Can you work these out from the drawing? Everything is in mm from the part's minimum corner. A direction names the side the tool comes from. Give positions to 0.01 mm unless a question says otherwise; leave off trailing zeros. Loops run counter-clockwise (first coordinate to the right, second up) from the corner with the lowest first, then second, coordinate; pieces in that order, holes last. Notation, with made-up numbers: (39.5, -6) - (85.5, -6) arc R14 ccw to (85.5, -1) - close; hole circle Ø9 at (-23.5, -3.5). An arc over 180 degrees is marked (long way). Write each question's results on one line, items separated by ' | '. Start each with the question number.
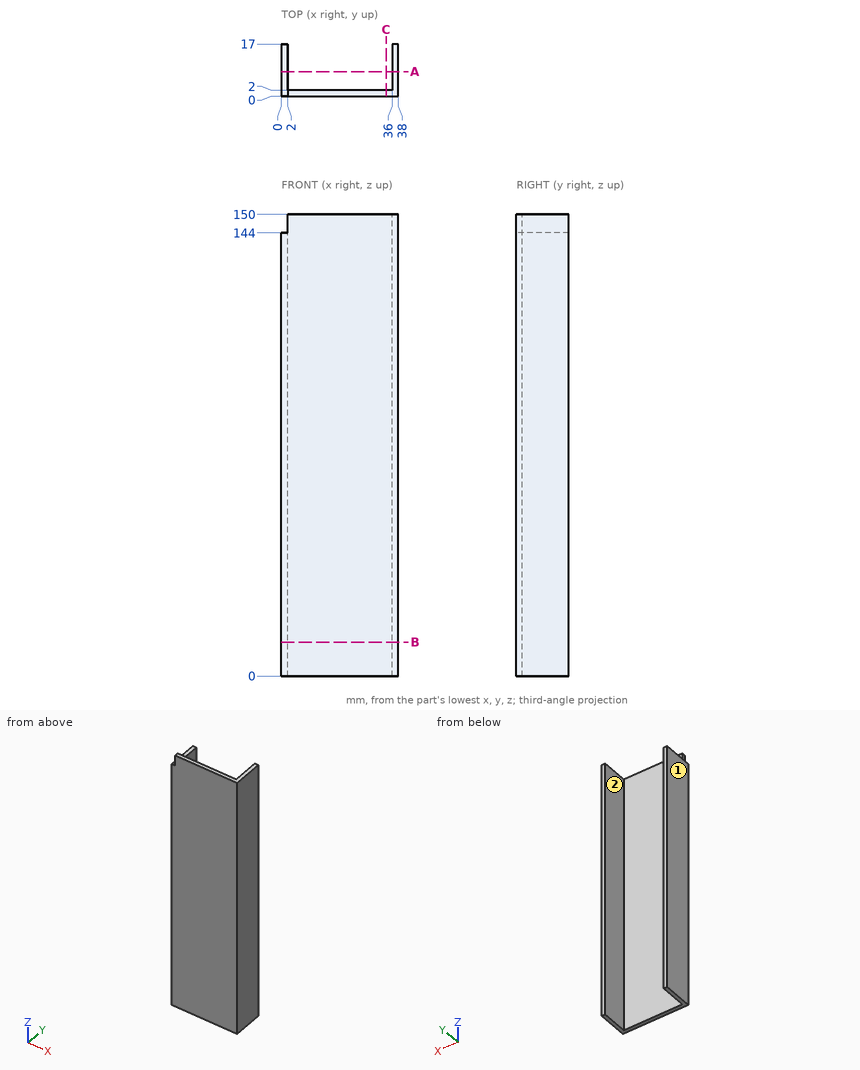
Q1. I want a section at C-C, the plane x = 34. List the corners of the cut face in (y, z) for me, then the cut area to 3 significant figures.
Q2. Which directions (+Z, -Z, +X, -X, +Y, -Y) give clear straight access to the entire face, cutting with the end or side of a thin tool? Please do the marked faces 1 and 2.
Q3. I want a section at A-A, the plane y = 8. List the corners of the cut face in (x, z) for me.
Q4. I want a section at B-B, the plane z = 11. List the corners of the cut face in (x, y) for me.
Q5. I need wall thicknesses on L1, parallel to X at y = 12.5, z = 111.5; L2, parallel to Y at x = 4.5, z = 143. Which ranges of each line are inside material? Lowest first, please. Write a range as from..to.
Q6. I'm going to push flat-ended pins straight in: pin 1 Ø1.5 at (x, z) = (28, 63) entering from +Y; pin 2 Ø10 at (x, y) = (21.5, 5.5) entering from -Z; pin 3 Ø0.6 at (y, z) = (1, 145.5) entering from -X; pin 4 Ø0.6 at (x, y) = (1.5, 8.5) entering from +Z. Where does each tip first touch, or does it pass through?
Conclusion:
1) outline: (0, 0) - (2, 0) - (2, 150) - (0, 150) - close | area: 300 mm^2
2) face 1: +Z, -Z, -X, +Y, -Y | face 2: +Z, -Z, +Y
3) outline: (0, 0) - (2, 0) - (2, 144) - (0, 144) - close; (36, 0) - (38, 0) - (38, 150) - (36, 150) - close
4) outline: (0, 0) - (38, 0) - (38, 17) - (36, 17) - (36, 2) - (2, 2) - (2, 17) - (0, 17) - close
5) L1: 0..2, 36..38 | L2: 0..2
6) pin 1: y = 2 | pin 2: z = 0 | pin 3: x = 2 | pin 4: z = 144
